from build123d import *

# Parameters (mm, degrees)
F1_DEPTH = 3.7
F2_R     = 0.508


with BuildPart() as f1:
    # F0 (on Top) → F1 (new body)
    with BuildSketch(Plane.XY):
        with BuildLine():
            Line((0, 20.689665), (0, 0))
            Line((0, 0), (137.16, 0))
            Line((137.16, 0), (137.16, 20.689665))
            ThreePointArc((137.16, 20.689665), (137.811787, 23.491961), (139.633343, 25.718982))
            Line((139.633343, 25.718982), (205.826443, 76.7414))
            ThreePointArc((205.826443, 76.7414), (206.253265, 78.156808), (205.051112, 79.017263))
            Line((205.051112, 79.017263), (73.782288, 79.017263))
            ThreePointArc((73.782288, 79.017263), (71.734565, 78.678031), (69.905631, 77.69658))
            Line((69.905631, 77.69658), (2.473343, 25.718982))
            ThreePointArc((2.473343, 25.718982), (0.651787, 23.491961), (0, 20.689665))
        make_face()
    extrude(amount=F1_DEPTH)

    # F2
    f2_edges = [f1.edges().sort_by_distance(p)[0] for p in [
        (68.58, 0, 3.7),
        (68.58, 0, 0),
        (0, 0, 1.85),
        (0, 10.344832, 3.7),
        (137.16, 10.344832, 0),
        (137.16, 0, 1.85),
    ]]
    fillet(f2_edges, radius=F2_R)


solid = f1.part
Verification items for the finished model (mm, model axes). Give positions to 0.01 mm unless a question says otherwise; leave off trailing zeros. Loops run counter-clockwise (first coordinate to the right, second up) from the corner with the lowest first, then second, coordinate; pieces in that order, holes last.
1. Go/stop test with flat-tipped pins: P1, Ø1.3, axis at y = 11, z = 2.5, coming from the +X side; P2, Ø1.5, axis at y = 37, z = 2.5, coming from the +X side; P3, Ø1, axis at y = 70, z = 2.5, coming from the +X side. Record where each tip stops, or that it passes through.
Derived:
P1: stops at x = 137.16
P2: stops at x = 155.24
P3: stops at x = 197.73
2. Cross-section at A-A on y = 16. Record the cut outline in (x, z), and give its area (3 significant figures).
Derived:
outline: (0, 0.51) arc R0.51 ccw to (0.51, 0) - (136.65, 0) arc R0.51 ccw to (137.16, 0.51) - (137.16, 3.19) arc R0.51 ccw to (136.65, 3.7) - (0.51, 3.7) arc R0.51 ccw to (0, 3.19) - close
area: 507 mm2
3. Material ranges on probe 1 along X at (y, z) = (8.5, 0.75); probe 2 along Y at (x, z) = (99.5, 0.3); probe 3 along Y at (x, z) = (158, 2.1), recorded low to high.
Derived:
probe 1: x = 0 to 137.16
probe 2: y = 0.04 to 78.97
probe 3: y = 39.88 to 79.02
4. Cross-section at B-B on z = 2.2. Record the cut outline in (x, y), and give its area (3 significant figures).
Derived:
outline: (0, 0.51) arc R0.51 ccw to (0.51, 0) - (136.65, 0) arc R0.51 ccw to (137.16, 0.51) - (137.16, 20.69) arc R6.35 cw to (139.63, 25.72) - (205.83, 76.74) arc R1.27 ccw to (205.05, 79.02) - (73.78, 79.02) arc R6.35 ccw to (69.91, 77.7) - (2.47, 25.72) arc R6.35 ccw to (0, 20.69) - close
area: 10,800 mm2
